Can you work these out from the model? Positions are in its coordinate system, mm. Give positions to 0.01 mm unless a question says otherwise; leave off trailing zeros. Write each loop counter-clockwise with the first axis right and the second up, starting at its lowest first coordinate (ties: lowest second). Pieces come first, ordered by that corner, then holes.
1. Suppose I cut it at D-D (y = -0.75). Give the number of separate pieces and of enclosed holes in the cut face, and give its area (3 significant figures).
2. I'm going to push a flat-ended pin straight in: pin 1 (4 mm diameter, centred on x = -298.45, z = 178.24, fed in from -Y). Where does the tip first touch, or does it pass through?
3. Suppose I cut it at A-A (z = -23.5). Please give me the cut outline in (x, y) (3 decimals).
4. Suppose I cut it at B-B (x = -208.5). Please give me the cut outline in (y, z), and give its area (3 significant figures).
5. If I drill on probe 1 along X at (y, z) = (-0.45, -6) (3 decimals); probe 2 along Z at (x, y) = (-298.45, 0); probe 3 along X at (y, z) = (-0.65, 101.5), over which ranges is the centre line in solid material (lowest first)?
6. Suppose I cut it at C-C (z = 82). Please give me the cut outline in (x, y), and give its area (3 significant figures).
```python
from build123d import *

# Parameters (mm, degrees)
F0_W     = 622.3
F0_H     = 530.225
F0_R     = 3.175
F1_DEPTH = 1.27
F2_W     = 6.35
F2_H     = 73.025
F2_H_2   = 36.5125
F2_R     = 2.579688
F3_DEPTH = 2.541


with BuildPart() as f1:
    # F0 (on Front) → F1 (new body, symmetric)
    with BuildSketch(Plane.XZ):
        Rectangle(F0_W, F0_H)
        with Locations((-298.45, -250.3805)):
            Circle(F0_R, mode=Mode.SUBTRACT)
        with BuildLine():
            Line((-250.825, 24.1935), (-250.825, 51.1175))
            Line((-250.825, 51.1175), (-28.575, 51.1175))
            Line((-28.575, 51.1175), (-28.575, 24.1935))
            Line((-28.575, 24.1935), (-25.4, 24.1935))
            ThreePointArc((-25.4, 24.1935), (-20.574, 19.3675), (-25.4, 14.5415))
            Line((-25.4, 14.5415), (-28.575, 14.5415))
            Line((-28.575, 14.5415), (-28.575, -166.3065))
            Line((-28.575, -166.3065), (-25.4, -166.3065))
            ThreePointArc((-25.4, -166.3065), (-20.574, -171.1325), (-25.4, -175.9585))
            Line((-25.4, -175.9585), (-28.575, -175.9585))
            Line((-28.575, -175.9585), (-28.575, -202.8825))
            Line((-28.575, -202.8825), (-250.825, -202.8825))
            Line((-250.825, -202.8825), (-250.825, -175.9585))
            Line((-250.825, -175.9585), (-254, -175.9585))
            ThreePointArc((-254, -175.9585), (-258.826, -171.1325), (-254, -166.3065))
            Line((-254, -166.3065), (-250.825, -166.3065))
            Line((-250.825, -166.3065), (-250.825, 14.5415))
            Line((-250.825, 14.5415), (-254, 14.5415))
            ThreePointArc((-254, 14.5415), (-258.826, 19.3675), (-254, 24.1935))
            Line((-254, 24.1935), (-250.825, 24.1935))
        make_face(mode=Mode.SUBTRACT)
        with Locations((0, -250.3805)):
            Circle(F0_R, mode=Mode.SUBTRACT)
        with Locations((298.45, -250.3805)):
            Circle(F0_R, mode=Mode.SUBTRACT)
        with BuildLine():
            Line((28.575, -202.8825), (28.575, -175.9585))
            Line((28.575, -175.9585), (25.4, -175.9585))
            ThreePointArc((25.4, -175.9585), (20.574, -171.1325), (25.4, -166.3065))
            Line((25.4, -166.3065), (28.575, -166.3065))
            Line((28.575, -166.3065), (28.575, 14.5415))
            Line((28.575, 14.5415), (25.4, 14.5415))
            ThreePointArc((25.4, 14.5415), (20.574, 19.3675), (25.4, 24.1935))
            Line((25.4, 24.1935), (28.575, 24.1935))
            Line((28.575, 24.1935), (28.575, 51.1175))
            Line((28.575, 51.1175), (250.825, 51.1175))
            Line((250.825, 51.1175), (250.825, 24.1935))
            Line((250.825, 24.1935), (254, 24.1935))
            ThreePointArc((254, 24.1935), (258.826, 19.3675), (254, 14.5415))
            Line((254, 14.5415), (250.825, 14.5415))
            Line((250.825, 14.5415), (250.825, -166.3065))
            Line((250.825, -166.3065), (254, -166.3065))
            ThreePointArc((254, -166.3065), (258.826, -171.1325), (254, -175.9585))
            Line((254, -175.9585), (250.825, -175.9585))
            Line((250.825, -175.9585), (250.825, -202.8825))
            Line((250.825, -202.8825), (28.575, -202.8825))
        make_face(mode=Mode.SUBTRACT)
        with Locations((-298.45, 127.4445)):
            Circle(F0_R, mode=Mode.SUBTRACT)
        with Locations((-298.45, 178.2445)):
            Circle(F0_R, mode=Mode.SUBTRACT)
        with Locations((298.45, 127.4445)):
            Circle(F0_R, mode=Mode.SUBTRACT)
        with Locations((0, 257.6195)):
            Circle(F0_R, mode=Mode.SUBTRACT)
        with Locations((298.45, 178.2445)):
            Circle(F0_R, mode=Mode.SUBTRACT)
    extrude(amount=F1_DEPTH, both=True)

    # F2 (on face) → F3 (cut, through all)
    with BuildSketch(Plane.XZ.offset(1.27)):
        with Locations((-174.625, 87.63)):
            Rectangle(F2_W, F2_H)
        with Locations((-104.775, 87.63)):
            Rectangle(F2_W, F2_H)
        with Locations((-104.775, -221.13875)):
            Rectangle(F2_W, F2_H_2)
        with Locations((-174.625, -221.13875)):
            Rectangle(F2_W, F2_H_2)
        with Locations((104.775, 87.63)):
            Rectangle(F2_W, F2_H)
        with Locations((174.625, -221.13875)):
            Rectangle(F2_W, F2_H_2)
        with Locations((174.625, 87.63)):
            Rectangle(F2_W, F2_H)
        with Locations((104.775, -221.13875)):
            Rectangle(F2_W, F2_H_2)
        with Locations((225.425, 176.2125)):
            Circle(F2_R)
        with Locations((-225.425, 176.2125)):
            Circle(F2_R)
        with Locations((76.2, 176.2125)):
            Circle(F2_R)
        with Locations((-76.2, 176.2125)):
            Circle(F2_R)
    extrude(amount=-F3_DEPTH, mode=Mode.SUBTRACT)


solid = f1.part
```
Checks:
1. separate pieces: 1
1. enclosed holes: 14
1. area: 213,000 mm2
2. pin 1: passes through
3. outline: (-311.15, -1.27) - (-250.825, -1.27) - (-250.825, 1.27) - (-311.15, 1.27) - close; (-28.575, -1.27) - (28.575, -1.27) - (28.575, 1.27) - (-28.575, 1.27) - close; (250.825, -1.27) - (311.15, -1.27) - (311.15, 1.27) - (250.825, 1.27) - close
4. outline: (-1.27, -265.11) - (1.27, -265.11) - (1.27, -202.88) - (-1.27, -202.88) - close; (-1.27, 51.12) - (1.27, 51.12) - (1.27, 265.11) - (-1.27, 265.11) - close
4. area: 702 mm2
5. probe 1: x = -311.15 to -250.825, -28.575 to 28.575, 250.825 to 311.15
5. probe 2: z = -265.11 to -253.56, -247.21 to 124.27, 130.62 to 175.07, 181.42 to 265.11
5. probe 3: x = -311.15 to -177.8, -171.45 to -107.95, -101.6 to 101.6, 107.95 to 171.45, 177.8 to 311.15
6. outline: (-311.15, -1.27) - (-177.8, -1.27) - (-177.8, 1.27) - (-311.15, 1.27) - close; (-171.45, -1.27) - (-107.95, -1.27) - (-107.95, 1.27) - (-171.45, 1.27) - close; (-101.6, -1.27) - (101.6, -1.27) - (101.6, 1.27) - (-101.6, 1.27) - close; (107.95, -1.27) - (171.45, -1.27) - (171.45, 1.27) - (107.95, 1.27) - close; (177.8, -1.27) - (311.15, -1.27) - (311.15, 1.27) - (177.8, 1.27) - close
6. area: 1,520 mm2
